Drawing for the job (mm, zero at the part's lowest x, y, z). A direction names the side the tool comes from. Round coordinates to 2 decimals unless told otherwise and drop trailing zeros. Order: outer loops, then holes, each group sorted by start corner. A loop starts at its lowest first (then second) coordinate and runs counter-clockwise, first axis right, second up. Notation, with made-up numbers: M 23,-20.75 L 28,-20.75 A15 cw 28,8.25 Z; hole C 22,53.25 d5. An arc over 180 degrees is marked long. One line per item, written item: value. Start each with the question number.
Item 1: Probe L1, parallel to Z at x = 40, y = 5.75; L2, parallel to Z at x = 40, y = 12.75; L3, parallel to X at y = 11.25, z = 70. List the from-to ranges inside material, lowest first.
Item 2: Band-saw the part on C-C, the plane y = 20.5. Write the cut outline in (x, z), then the cut area to 3 significant figures.
Item 3: Pin check, flat tips, straight feed: pin 1 (3 mm diameter, centred on x = 55, y = 20.5, fed in from -Z); pin 2 (5 mm diameter, centred on x = 32, y = 3, fed in from +Z); pin 3 (6 mm diameter, centred on x = 15.5, y = 15, fed in from -Z). Stop position of each tip, or through.
Item 4: Two-plate mould, pull along X, no slides. Class the marked faces 4, 5 and 6: +X half, -X half, draft (parallel to the pull), parting line (faces both ways), or undercut.
Item 5: Tool access for the marked faces 1, 2 and 3: list every direction of +Z, -Z, +X, -X, +Y, -Y with a clear straight run to the whole face (end or side of a thin tool).
Item 6: Band-saw the part on A-A, the plane z = 40. Write the cut outline in (x, y).
Item 7: Band-saw the part on D-D, the plane y = 11. Write the cut outline in (x, z), then the cut area to 3 significant figures.
Item 8: Band-saw the part on B-B, the plane y = 3.25. Write the cut outline in (x, z), then the cut area to 3 significant figures.
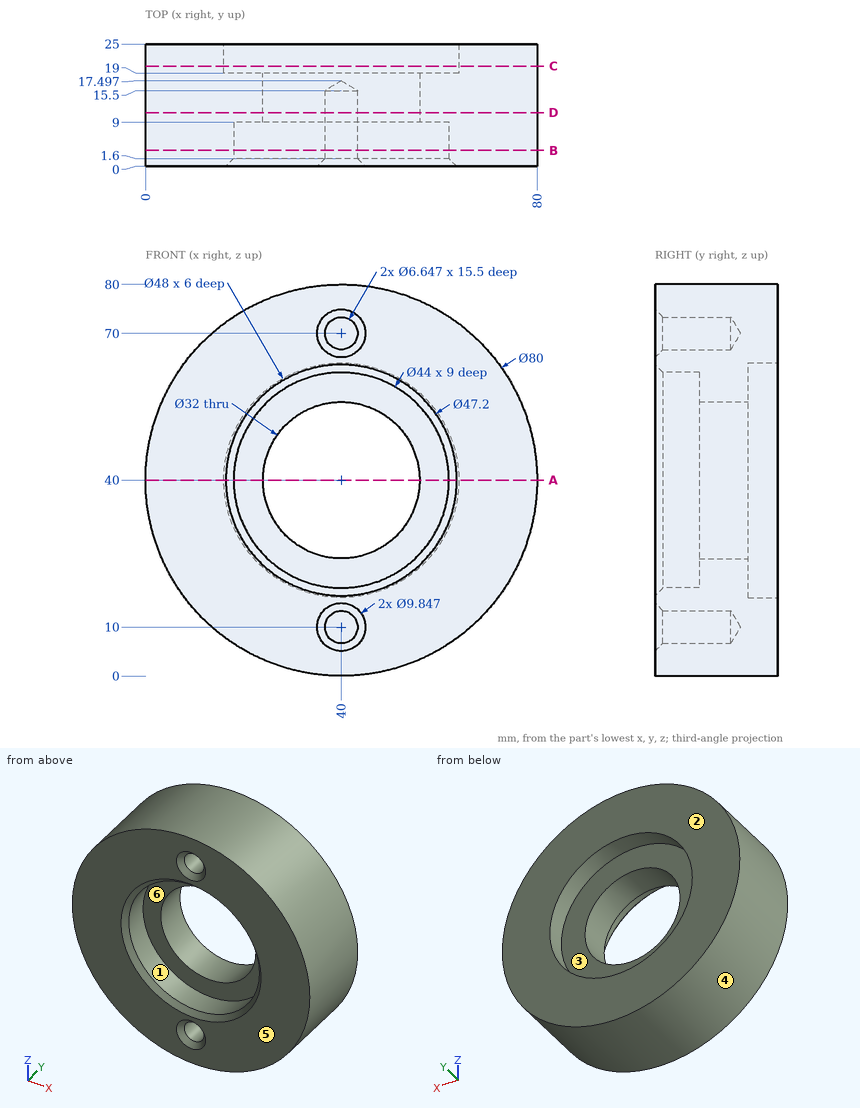
Output:
1. L1: z = 0 to 6.68, 13.32 to 18, 62 to 66.68, 73.32 to 80
1. L2: z = 0 to 6.68, 13.32 to 24, 56 to 66.68, 73.32 to 80
1. L3: x = 13.54 to 36.68, 43.32 to 66.46
2. outline: C 40,40 d80; hole C 40,40 d48
2. area: 3,220 mm²
3. pin 1: stops at z = 2.35
3. pin 2: stops at z = 79.62
3. pin 3: stops at z = 6.27
4. face 4: parting line
4. face 5: draft
4. face 6: undercut
5. face 1: -Y
5. face 2: +Z, -Z, +X, -X, +Y
5. face 3: +Y
6. outline: M 0,0 L 16.4,0 L 18,1.6 L 18,9 L 24,9 L 24,19 L 16,19 L 16,25 L 0,25 Z; M 56,9 L 62,9 L 62,1.6 L 63.6,0 L 80,0 L 80,25 L 64,25 L 64,19 L 56,19 Z
7. outline: C 40,40 d80; hole C 40,40 d32; hole C 40,10 d6.65; hole C 40,70 d6.65
7. area: 4,150 mm²
8. outline: C 40,40 d80; hole C 40,40 d44; hole C 40,10 d6.65; hole C 40,70 d6.65
8. area: 3,440 mm²
